from build123d import *

# Parameters (mm, degrees)
SKETCH1_W           = 13.2
SKETCH1_H           = 7.9
BOSS_EXTRUDE1_DEPTH = 9.5
SKETCH2_R           = 3
BOSS_EXTRUDE2_DEPTH = 8.8
SKETCH4_R           = 2.5
CUT_EXTRUDE1_DEPTH  = 2
SKETCH5_R           = 1.5
BOSS_EXTRUDE3_DEPTH = 13
REVOLVE2_ANGLE      = 180
FILLET1_R           = 1
SKETCH6_W           = 0.8
SKETCH6_H           = 2
BOSS_EXTRUDE4_DEPTH = 4
SKETCH7_W           = 1
SKETCH7_H           = 2
CUT_EXTRUDE3_DEPTH  = 32.795951
FILLET3_R           = 0.5


with BuildPart() as part:
    # Sketch1 → Boss-Extrude1 (new body)
    with BuildSketch(Plane(origin=(0, 0, 0), x_dir=(1, 0, 0), z_dir=(0, 1, 0))):
        Rectangle(SKETCH1_W, SKETCH1_H)
    extrude(amount=BOSS_EXTRUDE1_DEPTH)

    # Sketch2 → Boss-Extrude2 (add)
    with BuildSketch(Plane(origin=(0, 9.5, 0), x_dir=(1, 0, 0), z_dir=(0, 1, 0))):
        with Locations(Location((0, 0, 0), (0, 0, 270))):
            Circle(SKETCH2_R)
    extrude(amount=BOSS_EXTRUDE2_DEPTH)

    # Sketch4 → Cut-Extrude1 (cut)
    with BuildSketch(Plane(origin=(0, 18.3, 0), x_dir=(1, 0, 0), z_dir=(0, 1, 0))):
        with Locations(Location((0, 0, 0), (0, 0, 270))):
            Circle(SKETCH4_R)
    extrude(amount=-CUT_EXTRUDE1_DEPTH, mode=Mode.SUBTRACT)

    # Sketch5 → Boss-Extrude3 (add)
    with BuildSketch(Plane(origin=(0, 16.3, 0), x_dir=(1, 0, 0), z_dir=(0, 1, 0))):
        with Locations(Location((0, 0, 0), (0, 0, 90))):
            Circle(SKETCH5_R)
    extrude(amount=BOSS_EXTRUDE3_DEPTH)

    # Sketch3 → Revolve2 (revolve)
    with BuildSketch(Plane(origin=(0, 16.3, 0), x_dir=(1, 0, 0), z_dir=(0, 1, 0))):
        with BuildLine():
            Line((0, -2.5), (0, 2.5))
            ThreePointArc((0, 2.5), (-2.5, 0), (0, -2.5))
        make_face()
    revolve(axis=Axis((0, 16.3, 3), (0, 0, -1)), revolution_arc=REVOLVE2_ANGLE)

    # Fillet1
    fillet1_edges = [part.edges().sort_by_distance(p)[0] for p in [
        (0, 29.3, 1.5),
    ]]
    fillet(fillet1_edges, radius=FILLET1_R)

    # Sketch6 → Boss-Extrude4 (add)
    with BuildSketch(Plane.XZ):
        with Locations((-4.7, 0)):
            Rectangle(SKETCH6_W, SKETCH6_H)
        Rectangle(SKETCH6_W, SKETCH6_H)
    extrude(amount=BOSS_EXTRUDE4_DEPTH)

    # Sketch7 → Cut-Extrude3 (cut, through all)
    with BuildSketch(Plane.ZY.offset(5.1)):
        with Locations((0, -2.5)):
            Rectangle(SKETCH7_W, SKETCH7_H)
    extrude(amount=-CUT_EXTRUDE3_DEPTH, mode=Mode.SUBTRACT)

    # Fillet3
    fillet3_edges = [part.edges().sort_by_distance(p)[0] for p in [
        (0, -4, 1),
        (0, -4, -1),
        (-4.7, -4, -1),
        (-4.7, -4, 1),
        (0, -3.5, -0.5),
        (0, -1.5, -0.5),
        (0, -3.5, 0.5),
        (0, -1.5, 0.5),
        (-4.7, -1.5, 0.5),
        (-4.7, -1.5, -0.5),
        (-4.7, -3.5, 0.5),
        (-4.7, -3.5, -0.5),
    ]]
    fillet(fillet3_edges, radius=FILLET3_R - 0.0001)  # a hair under: the kernel refuses the full size


solid = part.part
Could you check a few things on this model? Use its own coordinates, in mm. A direction names the side the tool comes from. Give positions to 0.01 mm unless a question says otherwise; leave off trailing zeros. Order: outer loops, then holes, each group sorted by start corner. A loop starts at its lowest first (then second) coordinate and runs counter-clockwise, first axis right, second up.
Item 1: For faces 1 (the face through (-4.3, -1.5, -0.5)), 2 (the face through (0, -2.5, 0.5)), 3 (the face through (0.4, -1.5, -0.5)), 4 (the face through (-0.45, 23.23, -1.43)), which set-ups out of +Z, -Z, +X, -X, +Y, -Y let a thin tool reach every point of the face, with its end or its side?
Item 2: If we section it at A-A, the plane y = 17: Write out the boundary of the cut face in (x, z), plus the area to 3 significant figures.
Item 3: If we section it at B-B, the plane y = 21.5: Write out the boundary of the cut face in (x, z), plus the area to 3 significant figures.
Item 4: If we mould it in two halves opening along Y, with no side actions, what happens to faces 5 (the face through (1, 0, 0)), 6 (the face through (-4.7, -2.5, -0.5)), 7 (the face through (-5.1, -1.5, -0.5))? For each: pulls with the +Y half, pulls with the -Y half, needs draft (parallel to the pull), parting line crosses it, or undercut.
Item 5: I need wall thicknesses on line 1 (X direction, y = 17.9, z = 0); line 2 (Y direction, x = 3.25, z = 2); line 3 (X direction, y = 17.8, z = 0). Which ranges of each line are inside material? Lowest first, please.
Item 6: I'm going to push flat-ended pins straight in: pin 1 (4 mm diameter, centred on x = 2.5, z = 2.5, fed in from +Y); pin 2 (0.6 mm diameter, centred on x = -4.5, y = -2.5, fed in from -Z); pin 3 (1.6 mm diameter, centred on y = -2, z = -0.5, fed in from +X). Where does each tip first touch, or does it pass through?
Values:
1. face 1: +Z, -Z, -Y
1. face 2: +X, -X
1. face 3: +Z, -Z, +X, -Y
1. face 4: +Y
2. outline: circle Ø6 at (0, 0); circle Ø4.8 at (0, 0); hole circle Ø5 at (0, 0)
2. area: 26.7 mm2
3. outline: circle Ø3 at (0, 0)
3. area: 7.07 mm2
4. face 5: pulls with the -Y half
4. face 6: undercut
4. face 7: needs draft
5. line 1: x = -3 to -2.5, -1.92 to 1.92, 2.5 to 3
5. line 2: y = 0 to 9.5
5. line 3: x = -3 to -2.5, -2 to 2, 2.5 to 3
6. pin 1: stops at y = 18.3
6. pin 2: stops at z = -1
6. pin 3: stops at x = 0.4
